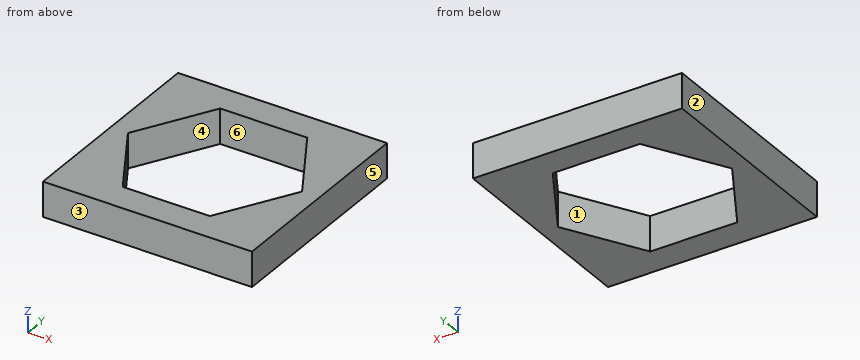
```python
from build123d import *

# Parameters (mm, degrees)
SCHIZZO1_W                   = 60
SCHIZZO1_H                   = 60
ESTRUSIONE_ESTRUSIONE1_DEPTH = 10


with BuildPart() as part:
    # Schizzo1 → Estrusione-Estrusione1 (new body)
    with BuildSketch(Plane.XY):
        Rectangle(SCHIZZO1_W, SCHIZZO1_H)
        Polygon((12.5, -21.650635095), (25, 0), (12.5, 21.650635095), (-12.5, 21.650635095), (-25, 0), (-12.5, -21.650635095), align=None, mode=Mode.SUBTRACT)
    extrude(amount=ESTRUSIONE_ESTRUSIONE1_DEPTH)


solid = part.part
```
Geometry check sheet. Reference: the model listing, model coordinates, mm. Face numbers are marked on the shaded views. A direction names the side the tool comes from. Give positions to 0.01 mm unless a question says otherwise; leave off trailing zeros. Order: outer loops, then holes, each group sorted by start corner. A loop starts at its lowest first (then second) coordinate and runs counter-clockwise, first axis right, second up. Notation, with made-up numbers: (6, 50.5) - (19, 50.5) arc R13 cw to (19, 61.5) - close; hole circle Ø3 at (-39.75, 23). An arc over 180 degrees is marked (long way). Write item = value, one per line. Start each with the question number.
1) Section check A-A (x = 7.5). Enter the section's corners in (y, z).
2) Draft check along X on the marked faces 1, 2, 3 and 4. Enter one of: released by +X, released by -X, zero draft, split by the parting line, or undercut.
3) Scan lines: L1, parallel to Y at x = 9, z = 2; L2, parallel to X at y = -1.5, z = 8.5; L3, parallel to X at y = 18.5, z = 3. Record each from-to range of solid material in increasing order.
4) Gauge pin test, flat end, axial feed: pin 1 Ø10 at (x, y) = (9.5, 14.5) entering from +Z. Record the tip position at first contact, or that the pin passes through.
5) Section check B-B (y = 3.5). Enter the section's corners in (x, z), then the cut area to 3 significant figures.
6) Section check C-C (z = 2). Enter the section's corners in (x, y).
7) Access from +Z, -Z, +X, -X, +Y, -Y to the whole of each face (thin tool, end or side, straight path). Record for the marked faces 5 and 6.
Geometry check:
q1.outline = (-30, 0) - (-21.65, 0) - (-21.65, 10) - (-30, 10) - close; (21.65, 0) - (30, 0) - (30, 10) - (21.65, 10) - close
q2.face_1 = undercut
q2.face_2 = released by -X
q2.face_3 = zero draft
q2.face_4 = undercut
q3.L1 = -30 to -21.65, 21.65 to 30
q3.L2 = -30 to -24.13, 24.13 to 30
q3.L3 = -30 to -14.32, 14.32 to 30
q4.pin_1 = through
q5.outline = (-30, 0) - (-22.98, 0) - (-22.98, 10) - (-30, 10) - close; (22.98, 0) - (30, 0) - (30, 10) - (22.98, 10) - close
q5.area = 140 mm2
q6.outline = (-30, -30) - (30, -30) - (30, 30) - (-30, 30) - close; hole (-25, 0) - (-12.5, -21.65) - (12.5, -21.65) - (25, 0) - (12.5, 21.65) - (-12.5, 21.65) - close
q7.face_5 = +Z, -Z, +X, +Y, -Y
q7.face_6 = +Z, -Z
